Check sheet for the modelled part. Datum: model origin and axes. Units: mm. Face numbers are marked on the shaded views. A direction names the side the tool comes from. Give positions to 0.01 mm unless a question says otherwise; leave off trailing zeros. Write each loop counter-clockwise with the first axis right and the second up, starting at its lowest first coordinate (ties: lowest second). Pieces come first, ordered by that corner, then holes. Notation, with made-up numbers: (58.25, 44.5) -> (107.25, 44.5) arc R23 ccw to (107.25, 54.5) -> close; hole circle Ø3 at (62, -28.5). An arc over 180 degrees is marked (long way). Answer as a JSON object with one key per item and string values.
Autodesk Inventor part; units mm, degrees
ref_plane "YZ Plane" through (0, 0, 0) normal (1, 0, 0) x (0, 1, 0)
ref_plane "XZ Plane" through (0, 0, 0) normal (0, 1, 0) x (-1, 0, 0)
ref_plane "XY Plane" through (0, 0, 0) normal (0, 0, 1) x (1, 0, 0)
sketch "Sketch1" plane through (0, 0, 0) normal (0, 1, 0) x (-1, 0, 0)
  line L0 (10.16, 0) -> (10.16, -36.068)
  line L1 (0, -36.068) -> (0, 0) construction
  circle A0 centre (5.08, -25.908) radius 2.9655
  line L2 (10.16, 0) -> (6.096, 0) construction
  line L3 (3.9775, 0) -> (0.0978, 0) construction
  line L4 (4.064, -3.81) -> (4.064, -14.8101) construction
  arc A1 (4.064, -14.8101) -> (6.096, -14.812) centre (5.0772, -17.8191) ccw
  line L5 (5.08, -31.75) -> (24.746, -31.75) construction
  line L6 (0, -4.7834) -> (2.794, -4.7834) construction
  line L7 (2.794, -4.7834) -> (2.794, -13.6734) construction
  line L8 (2.794, -13.6734) -> (0, -13.6734) construction
  line L9 (0, -13.6734) -> (0, -4.7834) construction
  line L10 (4.064, -4.7834) -> (0, -4.7834) construction
  line L11 (5.08, -31.75) -> (9.398, -31.75) construction
  line L12 (10.16, 0) -> (6.096, 0)
  line L13 (4.064, 0) -> (0, 0)
  line L14 (0, 0) -> (0, -36.068)
  line L15 (5.08, -36.068) -> (8.255, -36.068) construction
  line L16 (10.16, -36.068) -> (10.16, -39.243)
  line L17 (10.16, -39.243) -> (0, -39.243)
  line L18 (0, -39.243) -> (0, -36.068)
  line L19 (5.0772, -17.8191) -> (26.8769, -17.8191) construction
  arc A2 (4.064, -0.5428) -> (4.064, -1.7162) centre (4.307, -1.1295) ccw
  line L20 (4.064, -0.5428) -> (4.064, 0)
  arc A3 (4.064, -1.9422) -> (4.064, -3.5201) centre (4.307, -2.7311) ccw
  line L21 (4.064, -14.8101) -> (4.064, -3.5201)
  line L22 (4.064, -1.9422) -> (4.064, -1.7162)
  line L23 (4.064, -3.5201) -> (4.064, -3.81) construction
  line L24 (4.064, 0) -> (4.064, -0.5428) construction
  line L25 (4.064, -1.7162) -> (4.064, -1.9422) construction
  arc A4 (6.0904, -1.7162) -> (6.0904, -0.5428) centre (5.8475, -1.1295) ccw
  arc A5 (6.0904, -3.5201) -> (6.0904, -1.9422) centre (5.8475, -2.7311) ccw
  line L26 (6.096, -0.5451) -> (6.096, 0) construction
  line L27 (6.096, -3.5183) -> (6.096, -14.812)
  line L28 (6.096, 0) -> (6.096, -0.5451)
  line L29 (6.096, -1.7138) -> (6.096, -1.9439)
  line L30 (6.096, -3.81) -> (6.096, -3.5183) construction
  line L31 (6.096, -1.9439) -> (6.096, -1.7138) construction
  dimension "d0" = 10.16
  dimension "d3" = 5.9309
  dimension "d11" = 25.908
  dimension "d18" = 6.35
  dimension "d20" = 8.89
  dimension "d21" = 2.794
extrude "Extrusion1" add sketch "Sketch1" along normal blind 19.05
sketch "Sketch2" plane through (0, 0, 0) normal (1, 0, 0) x (0, 0, -1)
  line L0 (39.243, 0) -> (0, 0) construction
  line L1 (0, 19.05) -> (39.243, 19.05) construction
  line L2 (0, 0) -> (0, 19.05) construction
  line L3 (36.068, 9.525) -> (0, 9.525) construction
  line L4 (20.9941, 0) -> (14.812, 0) construction
  line L5 (3.81, 19.05) -> (14.812, 19.05) construction
  line L6 (14.6467, 0) -> (3.81, 0) construction
  line L7 (14.6467, 0) -> (14.6467, 19.05) construction
  line L8 (3.81, 19.05) -> (14.6467, 19.05) construction
  line L9 (3.81, 0) -> (3.81, 19.05) construction
  line L10 (14.6467, 9.525) -> (3.81, 9.525) construction
  circle A0 centre (9.2284, 9.525) radius 1.8542
  line L11 (39.243, 0) -> (39.243, 19.05)
  point P0 (14.8101, 0)
  dimension "d26" = 3.7084
extrude "Extrusion2" cut sketch "Sketch2" against normal blind 19.05
sketch "Sketch3" plane through (0, 19.05, 0) normal (0, 1, 0) x (1, 0, 0)
  line L0 (0, 11.0826) -> (0, 7.3742)
  point P0 (0, 0)
sketch "Sketch4" plane through (0, 0, 0) normal (1, 0, 0) x (0, 0, -1)
  circle A0 centre (9.2284, 9.525) radius 1.8542
  line L0 (39.243, 0) -> (0, 0)
  line L1 (0, 19.05) -> (39.243, 19.05)
  line L2 (0, 0) -> (0, 19.05)
  line L3 (14.3084, 9.525) -> (11.7684, 5.1256)
  line L4 (11.7684, 5.1256) -> (6.6884, 5.1256)
  line L5 (6.6884, 5.1256) -> (4.1484, 9.525)
  line L6 (4.1484, 9.525) -> (6.6884, 13.9244)
  line L7 (6.6884, 13.9244) -> (11.7684, 13.9244)
  line L8 (11.7684, 13.9244) -> (14.3084, 9.525)
  line L9 (39.243, 0) -> (39.243, 19.05)
  dimension "d30" = 10.16
extrude "Extrusion3" cut sketch "Sketch4" against normal blind 1.778 contours L3 L4 L5 L6 L7 L8
ref_plane "Work Plane1" through (0, 0, -33.528) normal (0, 0, -1) x (-1, 0, 0)
sketch "Sketch6" plane through (0, 0, -33.528) normal (0, 0, -1) x (-1, 0, 0)
  line L0 (0.508, 9.5571) -> (2.8218, 13.5005)
  line L1 (7.3938, 13.4684) -> (9.652, 9.4929)
  line L2 (2.8218, 13.5005) -> (7.3938, 13.4684)
  line L3 (0.508, 9.5571) -> (2.8218, 13.5005)
  line L4 (2.7662, 5.5816) -> (0.508, 9.5571)
  line L5 (7.3382, 5.5495) -> (2.7662, 5.5816)
  line L6 (9.652, 9.4929) -> (7.3382, 5.5495)
  circle A0 centre (5.1347, 9.4929) radius 4.5726
  circle A1 centre (5.1347, 9.4929) radius 1.8415
  point P0 (0, 0)
  dimension "d38" = 3.683
extrude "Extrusion5" cut sketch "Sketch6" along normal mid plane 12.7 contours A1
sketch "Sketch7" plane through (0, 0, 0) normal (1, 0, 0) x (0, 0, -1)
  line L0 (3.81, 19.05) -> (14.812, 19.05)
  circle A0 centre (9.2284, 18.3833) radius 1.27
  line L1 (0, 19.05) -> (39.243, 19.05)
  line L2 (6.8407, 19.05) -> (6.8407, 19.558)
  line L3 (6.8407, 19.05) -> (7.3487, 19.05) construction
  line L4 (7.3243, 18.5023) -> (7.3243, 18.3436)
  line L5 (7.3243, 18.5023) -> (7.4831, 18.5023) construction
  line L6 (22.9425, 19.05) -> (28.8734, 19.05)
  line L7 (28.8734, 0) -> (22.9425, 0)
  line L8 (28.8734, 0) -> (28.8734, 19.05)
  line L9 (28.8734, 9.525) -> (35.9855, 9.525)
  line L10 (35.9855, 9.525) -> (32.4294, 9.525)
  circle A1 centre (35.6044, 18.0788) radius 2.286
  line L11 (32.4294, 9.525) -> (32.4294, 7.6962)
  line L12 (32.4294, 7.6962) -> (32.4294, 4.5212)
  line L13 (28.8729, 7.6514) -> (39.243, 7.6514)
  line L14 (32.4294, 7.6962) -> (35.6044, 7.6962) construction
  line L15 (32.4294, 4.5212) -> (35.6044, 4.5212)
  point P0 (0, 0)
  point P1 (36.068, 19.05)
  point P2 (28.188, 9.4929)
  dimension "d41" = 2.54
  dimension "d42" = 0.508
  dimension "d43" = 90
  dimension "d46" = 0.1588
  dimension "d47" = 90
  dimension "d48" = 4.572
  dimension "d49" = 1.8288
  dimension "d56" = 3.175
  dimension "d57" = 90
  dimension "d58" = 3.175
  dimension "d59" = 90
extrude "Extrusion6" cut sketch "Sketch7" against normal blind 55.88 contours A0 L0 | A1 L1 | L1 A1 | L0 A0
sketch "Sketch8" plane through (0, 19.05, 0) normal (0, 1, 0) x (1, 0, 0)
  circle A0 centre (-5.08, 25.908) radius 4.191
  point P0 (0, 0)
  dimension "d50" = 8.382
extrude "Extrusion7" cut sketch "Sketch8" against normal blind 6.1214
fillet "Fillet1" radius 2.54 2 edges at (-6.096, 9.525, -14.812) (-4.064, 9.525, -14.8101)
sketch "Sketch9" plane through (-10.16, 0, -39.243) normal (-1, 0, 0) x (0, 0, 1)
  circle A0 centre (30.0146, 9.525) radius 2.0066
  point P0 (39.243, 0)
  dimension "d61" = 4.0132
extrude "Extrusion8" cut sketch "Sketch9" against normal blind 12.7
properties part number "Neuroprobeholdermagiger"
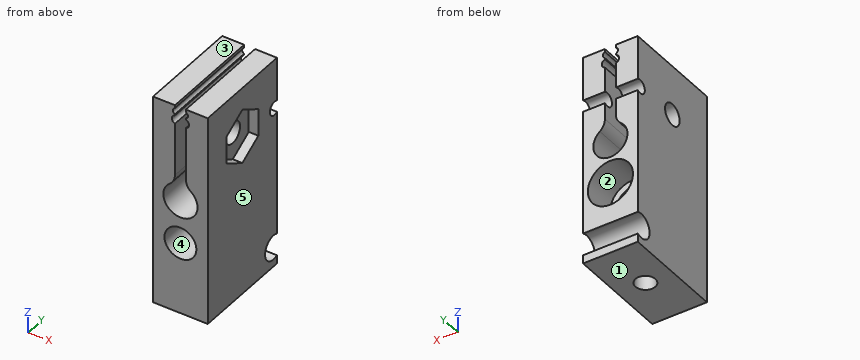
1. Sectioned sample at B-B, the plane z = -12.5. Enter the section's corners in (x, y), plus the area to 3 significant figures.
Determined:
{"outline": "(-10.16, 0) -> (-6.1, 0) -> (-6.1, 19.05) -> (-10.16, 19.05) -> close; (-4.06, 0) -> (0, 0) -> (0, 6.39) -> (-1.78, 6.39) -> (-1.78, 12.66) -> (0, 12.66) -> (0, 19.05) -> (-4.06, 19.05) -> close", "area": "144 mm^2"}
2. Sectioned sample at A-A, the plane x = -5.08. Enter the section's corners in (y, z), plus the area to 3 significant figures.
Determined:
{"outline": "(0, -39.24) -> (7.65, -39.24) -> (7.65, -28.87) -> (0, -28.87) -> close; (0, -22.94) -> (12.93, -22.94) -> (12.93, -21.72) -> (19.05, -21.72) -> (19.05, -20.99) -> (0, -20.99) -> close; (11.33, -39.24) -> (19.05, -39.24) -> (19.05, -37.67) arc R2.29 cw (long way) to (19.05, -33.53) -> (19.05, -30.1) -> (12.93, -30.1) -> (12.93, -28.87) -> (11.33, -28.87) -> close", "area": "169 mm^2"}
3. Access from +Z, -Z, +X, -X, +Y, -Y to the whole of each face (thin tool, end or side, straight path). Record for the marked faces 1 and 2.
Determined:
{"face 1": "-Z, +X, -X, +Y, -Y", "face 2": "+Y"}
4. Scan lines: L1, parallel to X at y = 14, z = -5.5; L2, parallel to Z at x = -2.75, y = 6.5; L3, parallel to Z at x = -5.08, y = 9.5. Record each from-to range of solid material in increasing order. Write a range as [from, to].
Determined:
{"L1": "[-10.16, -6.1], [-4.06, 0]", "L2": "[-39.24, -27.74], [-24.07, -19.98], [-15.66, 0]", "L3": "[-22.94, -20.99]"}
5. Sectioned sample at D-D, the plane z = -31.5. Enter the section's corners in (x, y), plus the area to 3 significant figures.
Determined:
{"outline": "(-10.16, 0) -> (0, 0) -> (0, 19.05) -> (-10.16, 19.05) -> close; hole circle Ø3.68 at (-5.13, 9.49)", "area": "183 mm^2"}
6. Mould release check, pull along X, two halves, no side actions. Record for the marked faces 3, 4 and 5: released by +X, released by -X, zero draft, split by the parting line, or undercut.
Determined:
{"face 3": "zero draft", "face 4": "undercut", "face 5": "released by +X"}
7. Go/stop test with flat-tipped pins: P1, Ø2.5, axis at y = 18.08, z = -35.6, coming from the +X side; P2, Ø0.5, axis at x = -0.5, z = -9, coming from the +Y side; P3, Ø3.5, axis at x = -5.13, y = 9.49, coming from the -Z side. Record where each tip stops, or that it passes through.
Determined:
{"P1": "through", "P2": "y = 17.21", "P3": "z = -23.55"}
